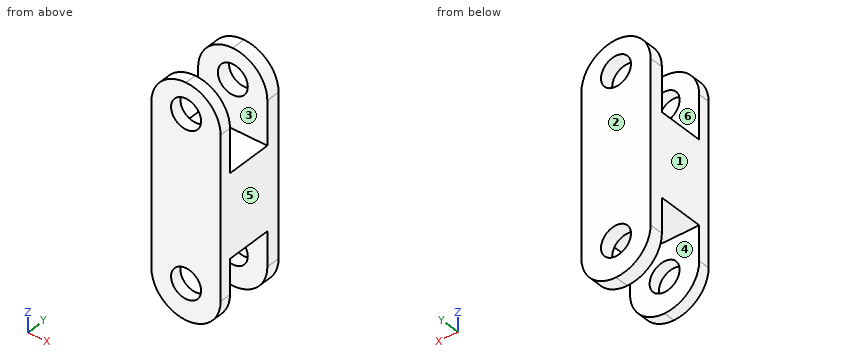
from build123d import *

# Parameters (mm, degrees)
SKETCH1_W               = 7.62
SKETCH1_H               = 25.4
EXTRUDE_THIN1_DEPTH     = 7.874
FILLET1_R               = 3.81
SKETCH3_R               = 1.651
CUT_EXTRUDE1_DEPTH      = 7.874
LPATTERN1_COUNT         = 2
LPATTERN1_PITCH         = 18.11528
SKETCH5_W               = 3.81
SKETCH5_H               = 5.08
CUT_EXTRUDE_THIN1_DEPTH = 60.226546789
CUT_EXTRUDE_THIN2_START = -7.874
SKETCH5_3_W             = 5.08
SKETCH5_3_H             = 5.08
CUT_EXTRUDE_THIN2_DEPTH = 68.100546789
LPATTERN2_COUNT         = 2
LPATTERN2_PITCH         = 18.034
LPATTERN4_COUNT         = 2
LPATTERN4_PITCH         = 18.034


with BuildPart() as part:
    # Sketch1 → Extrude-Thin1 (new body)
    with BuildSketch(Plane(origin=(0, 0, 0), x_dir=(1, 0, 0), z_dir=(0, 1, 0))):
        with Locations((-3.81, -45.504119859)):
            Rectangle(SKETCH1_W, SKETCH1_H)
    extrude(amount=EXTRUDE_THIN1_DEPTH)

    # Fillet1
    fillet1_edges = [part.edges().sort_by_distance(p)[0] for p in [
        (-7.62, 3.937, 32.804119859),
        (0, 3.937, 32.804119859),
        (0, 3.937, 58.204119859),
        (-7.62, 3.937, 58.204119859),
    ]]
    fillet(fillet1_edges, radius=FILLET1_R - 0.0001)  # a hair under: the kernel refuses the full size

    # Sketch3 → Cut-Extrude1 (cut)
    with BuildSketch(Plane(origin=(0, 7.874, 0), x_dir=(1, 0, 0), z_dir=(0, 1, 0))):
        with Locations(Location((-3.805586637, -54.841580585, 0), (0, 0, 270))):
            Circle(SKETCH3_R)
    cut_extrude1 = extrude(amount=-CUT_EXTRUDE1_DEPTH, mode=Mode.SUBTRACT)

    # LPattern1: Cut-Extrude1 ×2
    with Locations(*[(0, 0, -i * LPATTERN1_PITCH) for i in range(1, LPATTERN1_COUNT)]):
        add(cut_extrude1, mode=Mode.SUBTRACT)

    # Sketch5 → Cut-Extrude-Thin1 (cut, symmetric)
    with BuildSketch(Plane(origin=(0, 0, 0), x_dir=(0, 0, -1), z_dir=(1, 0, 0))):
        with Locations((-38.519119859, 3.808272384)):
            Rectangle(SKETCH5_W, SKETCH5_H)
    cut_extrude_thin1 = extrude(amount=CUT_EXTRUDE_THIN1_DEPTH, both=True, mode=Mode.SUBTRACT)

    # Sketch5<3> → Cut-Extrude-Thin2 (cut)
    with BuildSketch(Plane(origin=(0, 0, 0), x_dir=(0, 0, -1), z_dir=(1, 0, 0)).offset(CUT_EXTRUDE_THIN2_START)):
        with Locations((-34.074119859, 3.808272384)):
            Rectangle(SKETCH5_3_W, SKETCH5_3_H)
    cut_extrude_thin2 = extrude(amount=CUT_EXTRUDE_THIN2_DEPTH, mode=Mode.SUBTRACT)

    # LPattern2: Cut-Extrude-Thin2 ×2
    with Locations(*[(0, 0, i * LPATTERN2_PITCH) for i in range(1, LPATTERN2_COUNT)]):
        add(cut_extrude_thin2, mode=Mode.SUBTRACT)

    # LPattern4: Cut-Extrude-Thin1 ×2
    with Locations(*[(0, 0, i * LPATTERN4_PITCH) for i in range(1, LPATTERN4_COUNT)]):
        add(cut_extrude_thin1, mode=Mode.SUBTRACT)


solid = part.part
Input: part model. Units: mm. Frame: model coordinates. Face numbers are marked on the shaded views. A direction names the side the tool comes from. Round coordinates to 2 decimals unless told otherwise and drop trailing zeros. Write each loop counter-clockwise with the first axis right and the second up, starting at its lowest first coordinate (ties: lowest second). Pieces come first, ordered by that corner, then holes.
1) Cut plane D-D (y = 7.5). Count the separate pieces of the cut face and the enclosed holes in it, then the cut area to 3 significant figures.
2) Ray query, L1, parallel to Z at x = -3.75, y = 1; L2, parallel to Y at x = -2.75, z = 56.75; L3, parallel to Z at x = -3.25, y = 7.5. Return the intervals inside material, ascending.
3) Draft query along Y for the marked faces 1, 2 and 3. Return one class per face: pulls with the +Y half, pulls with the -Y half, needs draft (parallel to the pull), parting line crosses it, or undercut.
4) Cut plane C-C (z = 35.75). Return the cut outline in (x, y).
5) Reachability of the marked faces 4, 5 and 6 from +Z, -Z, +X, -X, +Y, -Y: full face, straight path, thin tool, end or side. Return the list, or none.
6) Cut plane B-B (x = -4.25). Return the cut outline in (y, z).
7) Contact query for flat-ended pins moving along their axis: P1, Ø2.5, axis at x = -3.81, z = 36.73, coming from the +Y side; P2, Ø4, axis at x = -2.5, y = 3, coming from the -Z side; P3, Ø1.5, axis at x = -3, y = 4, coming from the +Z side. Output: stop coordinate, or through.
8) Cut plane A-A (z = 50). Return the cut outline in (x, y).
Geometry says:
1. separate pieces: 1
1. enclosed holes: 2
1. area: 164 mm2
2. L1: z = 32.8 to 35.08, 38.38 to 53.19, 56.49 to 58.2
2. L2: y = 0 to 1.27, 6.35 to 7.87
2. L3: z = 32.85 to 35.17, 38.28 to 53.29, 56.4 to 58.16
3. face 1: needs draft
3. face 2: pulls with the +Y half
3. face 3: undercut
4. outline: (-7.52, 0) - (-5.14, 0) - (-5.14, 1.27) - (-7.52, 1.27) - close; (-7.52, 6.35) - (-5.14, 6.35) - (-5.14, 7.87) - (-7.52, 7.87) - close; (-2.47, 0) - (-0.1, 0) - (-0.1, 1.27) - (-2.47, 1.27) - close; (-2.47, 6.35) - (-0.1, 6.35) - (-0.1, 7.87) - (-2.47, 7.87) - close
5. face 4: -Z, +X, -X
5. face 5: +Z, -Z, +X, +Y, -Y
5. face 6: +Z, +X, -X
6. outline: (0, 32.83) - (1.27, 32.83) - (1.27, 35.14) - (0, 35.14) - close; (0, 38.32) - (1.27, 38.32) - (1.27, 40.42) - (6.35, 40.42) - (6.35, 38.32) - (7.87, 38.32) - (7.87, 53.25) - (6.35, 53.25) - (6.35, 49.57) - (1.27, 49.57) - (1.27, 53.25) - (0, 53.25) - close; (0, 56.43) - (1.27, 56.43) - (1.27, 58.18) - (0, 58.18) - close; (6.35, 32.83) - (7.87, 32.83) - (7.87, 35.14) - (6.35, 35.14) - close; (6.35, 56.43) - (7.87, 56.43) - (7.87, 58.18) - (6.35, 58.18) - close
7. P1: passes through
7. P2: stops at z = 32.82
7. P3: stops at z = 49.57
8. outline: (-7.62, 0) - (0, 0) - (0, 1.27) - (-7.62, 1.27) - close; (-7.62, 6.35) - (0, 6.35) - (0, 7.87) - (-7.62, 7.87) - close
